Design review of the part built by this model. Coordinates are the model's own, in mm. A direction names the side the tool comes from. Coordinates: 2 decimals unless noted, no trailing zeros. Write each loop counter-clockwise with the first axis right and the second up, starting at its lowest first coordinate (ties: lowest second). Pieces come first, ordered by that corner, then holes. Notation, with made-up numbers: (-11.75, 75) - (8.25, 75) arc R21 cw to (8.25, 85) - close; hole circle Ø10 at (-34, 25.25). An arc over 180 degrees is marked (long way). One line per item, written item: value.
from build123d import *

# Parameters (mm, degrees)
SZKIC1_W                    = 75
SZKIC1_H                    = 75
DODANIE_WYCI_GNI_CIE1_DEPTH = 10
ZAOKR_GLENIE1_R             = 5
WYTNIJ_WYCI_GNI_CIE1_DEPTH  = 8
WYTNIJ_WYCI_GNI_CIE2_DEPTH  = 4
SZKIC7_R                    = 1.9
SZKIC7_R_2                  = 0.9
SZKIC7_R_3                  = 1.900523095
SZKIC7_R_4                  = 0.900523095
DODANIE_WYCI_GNI_CIE2_DEPTH = 8.7
SZKIC9_R                    = 0.900523095
SZKIC9_R_2                  = 0.9
DODANIE_WYCI_GNI_CIE3_DEPTH = 1
SZKIC10_R                   = 1.7
DODANIE_WYCI_GNI_CIE4_DEPTH = 1
SZKIC11_R                   = 2.45
SZKIC11_R_2                 = 1.7
DODANIE_WYCI_GNI_CIE5_DEPTH = 8.5
SZKIC19_W                   = 9
SZKIC19_H                   = 1.5
WYTNIJ_WYCI_GNI_CIE15_DEPTH = 10
SZKIC22_W                   = 4
SZKIC22_H                   = 1
DODANIE_WYCI_GNI_CIE6_DEPTH = 0.3
SZKIC24_W                   = 4
SZKIC24_H                   = 1
DODANIE_WYCI_GNI_CIE7_DEPTH = 0.3
WYTNIJ_WYCI_GNI_CIE13_DEPTH = 55
WYTNIJ_WYCI_GNI_CIE14_DEPTH = 55


with BuildPart() as part:
    # Szkic1 → Dodanie-wyciągnięcie1 (new body)
    with BuildSketch(Plane(origin=(0, 0, 0), x_dir=(1, 0, 0), z_dir=(0, 1, 0))):
        with Locations((37.5, 37.5)):
            Rectangle(SZKIC1_W, SZKIC1_H)
    extrude(amount=DODANIE_WYCI_GNI_CIE1_DEPTH)

    # Zaokrąglenie1
    zaokr_glenie1_edges = [part.edges().sort_by_distance(p)[0] for p in [
        (0, 5, 0),
        (0, 5, -75),
        (75, 5, -75),
        (75, 5, 0),
    ]]
    fillet(zaokr_glenie1_edges, radius=ZAOKR_GLENIE1_R)

    # Szkic4 → Wytnij-wyciągnięcie1 (cut)
    with BuildSketch(Plane(origin=(0, 10, 0), x_dir=(1, 0, 0), z_dir=(0, 1, 0))):
        with BuildLine():
            Line((2, 70), (2, 5))
            ThreePointArc((2, 5), (2.878679656, 2.878679656), (5, 2))
            Line((5, 2), (70, 2))
            ThreePointArc((70, 2), (72.121320344, 2.878679656), (73, 5))
            Line((73, 5), (73, 70))
            ThreePointArc((73, 70), (72.121320344, 72.121320344), (70, 73))
            Line((70, 73), (5, 73))
            ThreePointArc((5, 73), (2.878679656, 72.121320344), (2, 70))
        make_face()
    extrude(amount=-WYTNIJ_WYCI_GNI_CIE1_DEPTH, mode=Mode.SUBTRACT)

    # Szkic6 → Wytnij-wyciągnięcie2 (cut)
    with BuildSketch(Plane(origin=(0, 10, 0), x_dir=(1, 0, 0), z_dir=(0, 1, 0))):
        with BuildLine():
            Line((1, 70), (1, 5))
            ThreePointArc((1, 5), (2.171572875, 2.171572875), (5, 1))
            Line((5, 1), (70, 1))
            ThreePointArc((70, 1), (72.828427125, 2.171572875), (74, 5))
            Line((74, 5), (74, 70))
            ThreePointArc((74, 70), (72.828427125, 72.828427125), (70, 74))
            Line((70, 74), (5, 74))
            ThreePointArc((5, 74), (2.171572875, 72.828427125), (1, 70))
        make_face()
        with BuildLine():
            Line((2, 70), (2, 5))
            ThreePointArc((2, 5), (2.878679656, 2.878679656), (5, 2))
            Line((5, 2), (70, 2))
            ThreePointArc((70, 2), (72.121320344, 2.878679656), (73, 5))
            Line((73, 5), (73, 70))
            ThreePointArc((73, 70), (72.121320344, 72.121320344), (70, 73))
            Line((70, 73), (5, 73))
            ThreePointArc((5, 73), (2.878679656, 72.121320344), (2, 70))
        make_face(mode=Mode.SUBTRACT)
    extrude(amount=-WYTNIJ_WYCI_GNI_CIE2_DEPTH, mode=Mode.SUBTRACT)

    # Szkic7 → Dodanie-wyciągnięcie2 (add)
    with BuildSketch(Plane(origin=(0, 2, 0), x_dir=(1, 0, 0), z_dir=(0, 1, 0))):
        with Locations((24, 52)):
            Circle(SZKIC7_R)
        with Locations((24, 52)):
            Circle(SZKIC7_R_2, mode=Mode.SUBTRACT)
        with Locations((35.5, 52)):
            Circle(SZKIC7_R_3)
        with Locations((35.5, 52)):
            Circle(SZKIC7_R_4, mode=Mode.SUBTRACT)
        with Locations((35.5, 5)):
            Circle(SZKIC7_R)
        with Locations((35.5, 5)):
            Circle(SZKIC7_R_2, mode=Mode.SUBTRACT)
        with Locations((24, 5)):
            Circle(SZKIC7_R)
        with Locations((24, 5)):
            Circle(SZKIC7_R_2, mode=Mode.SUBTRACT)
    extrude(amount=DODANIE_WYCI_GNI_CIE2_DEPTH)

    # Szkic9 → Dodanie-wyciągnięcie3 (add)
    with BuildSketch(Plane(origin=(0, 2, 0), x_dir=(1, 0, 0), z_dir=(0, 1, 0))):
        with Locations((35.5, 52)):
            Circle(SZKIC9_R)
        with Locations((35.5, 5)):
            Circle(SZKIC9_R_2)
        with Locations((24, 5)):
            Circle(SZKIC9_R_2)
        with Locations((24, 52)):
            Circle(SZKIC9_R_2)
    extrude(amount=DODANIE_WYCI_GNI_CIE3_DEPTH)

    # Szkic10 → Dodanie-wyciągnięcie4 (add)
    with BuildSketch(Plane(origin=(0, 2, 0), x_dir=(1, 0, 0), z_dir=(0, 1, 0))):
        with Locations((67, 17)):
            Circle(SZKIC10_R)
        with Locations((67, 8)):
            Circle(SZKIC10_R)
    extrude(amount=DODANIE_WYCI_GNI_CIE4_DEPTH)

    # Szkic11 → Dodanie-wyciągnięcie5 (add)
    with BuildSketch(Plane(origin=(0, 2, 0), x_dir=(1, 0, 0), z_dir=(0, 1, 0))):
        with Locations((67, 17)):
            Circle(SZKIC11_R)
        with Locations((67, 17)):
            Circle(SZKIC11_R_2, mode=Mode.SUBTRACT)
        with Locations((67, 8)):
            Circle(SZKIC11_R)
        with Locations((67, 8)):
            Circle(SZKIC11_R_2, mode=Mode.SUBTRACT)
    extrude(amount=DODANIE_WYCI_GNI_CIE5_DEPTH)

    # Szkic19 → Wytnij-wyciągnięcie15 (cut)
    with BuildSketch(Plane(origin=(0, 0, -2), x_dir=(-1, 0, 0), z_dir=(0, 0, -1))):
        with Locations((-29.75, 9.25)):
            Rectangle(SZKIC19_W, SZKIC19_H)
    extrude(amount=-WYTNIJ_WYCI_GNI_CIE15_DEPTH, mode=Mode.SUBTRACT)

    # Szkic22 → Dodanie-wyciągnięcie6 (add)
    with BuildSketch(Plane.ZY.offset(-74)):
        with Locations((-37.5, 9.5)):
            Rectangle(SZKIC22_W, SZKIC22_H)
        with Locations((-63, 9.5)):
            Rectangle(SZKIC22_W, SZKIC22_H)
        with Locations((-12, 9.5)):
            Rectangle(SZKIC22_W, SZKIC22_H)
    extrude(amount=DODANIE_WYCI_GNI_CIE6_DEPTH)

    # Szkic24 → Dodanie-wyciągnięcie7 (add)
    with BuildSketch(Plane(origin=(1, 0, 0), x_dir=(0, 0, -1), z_dir=(1, 0, 0))):
        with Locations((12, 9.5)):
            Rectangle(SZKIC24_W, SZKIC24_H)
        with Locations((63, 9.5)):
            Rectangle(SZKIC24_W, SZKIC24_H)
        with Locations((37.5, 9.5)):
            Rectangle(SZKIC24_W, SZKIC24_H)
    extrude(amount=DODANIE_WYCI_GNI_CIE7_DEPTH)

    # Szkic25 → Wytnij-wyciągnięcie13 (cut)
    with BuildSketch(Plane.XY.offset(-10)):
        Polygon((1, 10), (1.3, 9.5), (1.3, 10), align=None)
    extrude(amount=-WYTNIJ_WYCI_GNI_CIE13_DEPTH, mode=Mode.SUBTRACT)

    # Szkic26 → Wytnij-wyciągnięcie14 (cut)
    with BuildSketch(Plane(origin=(0, 0, -65), x_dir=(-1, 0, 0), z_dir=(0, 0, -1))):
        Polygon((-74, 10), (-73.7, 10), (-73.7, 9.5), align=None)
    extrude(amount=-WYTNIJ_WYCI_GNI_CIE14_DEPTH, mode=Mode.SUBTRACT)


with BuildPart() as body_2:
    # Lustro5: mirrored copy
    add(part.part.mirror(Plane.ZX.offset(-10)))


solid = body_2.part
1. Mouldability with a two-part tool opening along X and no side actions: class faces 1 (the face through (24, -23, -52)), 2 (the face through (37, -20, -38)), 3 (the face through (73, -25, -1)), 4 (the face through (72.859, -28.028, -72.797)) as released by +X, released by -X, zero draft, split by the parting line, or undercut.
Answer block:
face 1: undercut
face 2: zero draft
face 3: released by +X
face 4: undercut
2. Consider section C-C, the plane x = 24. Write out the cut boundary in (y, z), then the cut area to 3 significant figures.
Answer block:
outline: (-30.7, -53.9) - (-22, -53.9) - (-22, -73) - (-26, -73) - (-26, -74) - (-30, -74) - (-30, -75) - (-20, -75) - (-20, 0) - (-30, 0) - (-30, -1) - (-26, -1) - (-26, -2) - (-22, -2) - (-22, -3.1) - (-30.7, -3.1) - (-30.7, -4.1) - (-23, -4.1) - (-23, -5.9) - (-30.7, -5.9) - (-30.7, -6.9) - (-22, -6.9) - (-22, -50.1) - (-30.7, -50.1) - (-30.7, -51.1) - (-23, -51.1) - (-23, -52.9) - (-30.7, -52.9) - close
area: 212 mm^2
3. Wall thickness on line 1 along Z through (x, y) = (24, -29); line 2 along X through (y, z) = (-25.75, -52); line 3 along Z through (x, y) = (67, -26.25): over which ranges is each line inside the solid? List them lowest first.
Answer block:
line 1: z = -75 to -74, -53.9 to -52.9, -51.1 to -50.1, -6.9 to -5.9, -4.1 to -3.1, -1 to 0
line 2: x = 0 to 2, 22.1 to 23.1, 24.9 to 25.9, 33.6 to 34.6, 36.4 to 37.4, 73 to 75
line 3: z = -75 to -74, -19.45 to -18.7, -15.3 to -14.55, -10.45 to -9.7, -6.3 to -5.55, -1 to 0
4. Consider section B-B, the plane z = -17. Write out the cut boundary in (x, y).
Answer block:
outline: (0, -30) - (1, -30) - (1, -26) - (2, -26) - (2, -22) - (64.55, -22) - (64.55, -30.5) - (65.3, -30.5) - (65.3, -23) - (68.7, -23) - (68.7, -30.5) - (69.45, -30.5) - (69.45, -22) - (73, -22) - (73, -26) - (74, -26) - (74, -30) - (75, -30) - (75, -20) - (0, -20) - close
5. For faces 5 (the face through (36, -30.7, -4)), 6 (the face through (35.088, -26.289, -50.145)), list the 3-axis set-ups (+Z, -Z, +X, -X, +Y, -Y) from which the entire face can be reached by the end or side of a thin tool; tool diameter is ignored.
Answer block:
face 5: +Z, -Z, +X, -X, -Y
face 6: -Y
6. Consider section D-D, the plane z = -60. Write out the cut boundary in (x, y), then the cut area to 3 significant figures.
Answer block:
outline: (0, -30) - (1, -30) - (1, -26) - (2, -26) - (2, -22) - (73, -22) - (73, -26) - (74, -26) - (74, -30) - (75, -30) - (75, -20) - (0, -20) - close
area: 174 mm^2
7. Insertion check: pin 1 Ø1 at (x, z) = (67.5, -17) entering from -Y; pin 2 Ø12 at (x, z) = (37.5, -17) entering from -Y. Each pin has a flat end and moves straight along its axis. Give the tip position at first contact, or say it passes through.
Answer block:
pin 1: stops at y = -23
pin 2: stops at y = -22
8. Consider section A-A, the plane x = 52. Write out the cut boundary in (y, z), then the cut area to 3 significant figures.
Answer block:
outline: (-30, -75) - (-20, -75) - (-20, 0) - (-30, 0) - (-30, -1) - (-26, -1) - (-26, -2) - (-22, -2) - (-22, -73) - (-26, -73) - (-26, -74) - (-30, -74) - close
area: 174 mm^2
